Check sheet for the drawn part. Datum: minimum x, y, z corner. Units: mm. Coordinates: 2 decimals unless noted, no trailing zeros. Order: outer loops, then holes, each group sorted by start corner. A loop starts at its lowest first (then second) coordinate and runs counter-clockwise, first axis right, second up. Notation, with made-up numbers: (4.5, 30) - (41.5, 30) arc R24 ccw to (41.5, 50) - close; hole circle Ø1 at (-8, -13). An arc over 180 degrees is marked (long way). Answer as CSV lines item,"result". Start each with the question number.
1. Section check C-C (z = 0.65). Record the cut outline in (x, y) (1 decimal).
2. Go/stop test with a flat-tipped pin: pin 1 (4 mm diameter, centred on x = 33.655, y = 64.77, fed in from -Z). Record where the tip stops, or that it passes through.
3. Section check B-B (x = 33.5). Record the cut outline in (y, z).
4. Section check A-A (y = 24.13). Record the cut outline in (x, z).
5. Material ranges on L1, parallel to X at y = 153.67, z = 0.65; L2, parallel to Y at x = 32, z = 0.45; L3, parallel to Y at x = 15, z = 0.5 (1 decimal), recorded low to high. Write a range as [from, to].
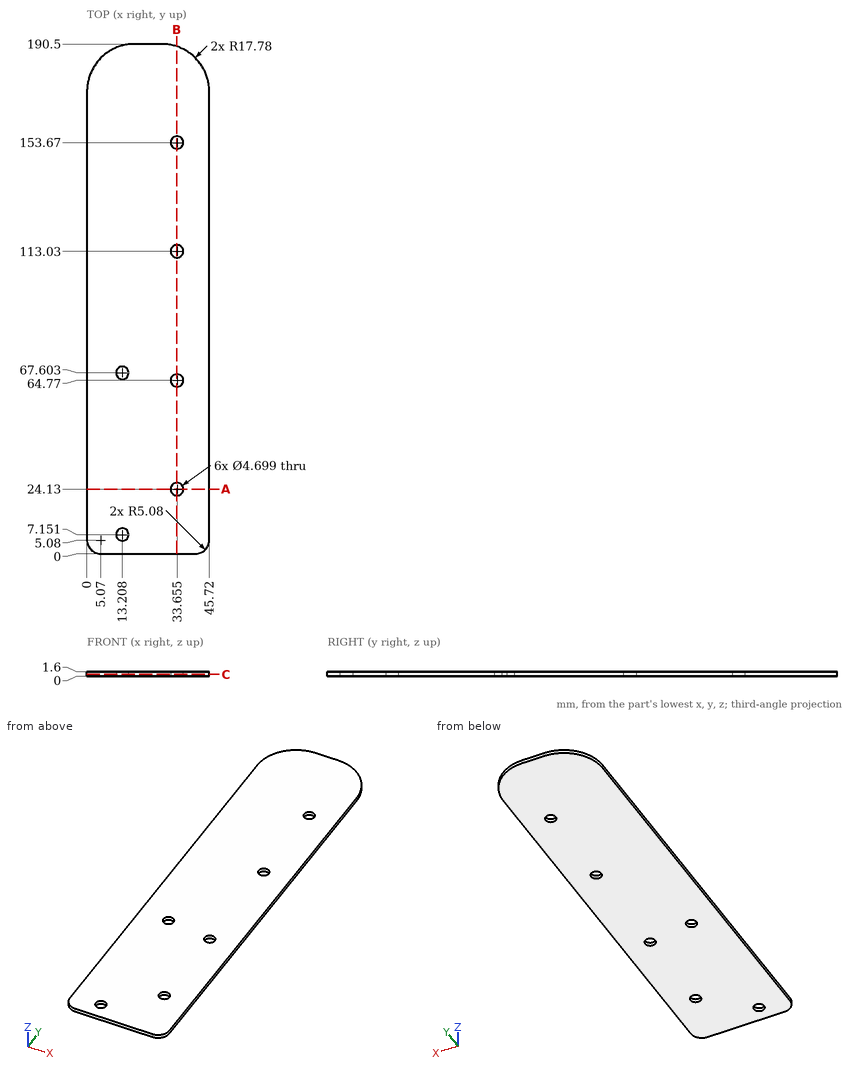
Evaluation:
1,outline,"(0, 4.8) arc R5.1 ccw to (5.1, 0) - (40.6, 0) arc R5.1 ccw to (45.7, 5.1) - (45.7, 172.7) arc R17.8 ccw to (27.9, 190.5) - (17.8, 190.5) arc R17.8 ccw to (0, 172.7) - close; hole circle Ø4.7 at (13.2, 7.2); hole circle Ø4.7 at (13.2, 67.6); hole circle Ø4.7 at (33.7, 24.1); hole circle Ø4.7 at (33.7, 64.8); hole circle Ø4.7 at (33.7, 113); hole circle Ø4.7 at (33.7, 153.7)"
2,pin 1,"passes through"
3,outline,"(0, 0) - (21.79, 0) - (21.79, 1.6) - (0, 1.6) - close; (26.47, 0) - (62.43, 0) - (62.43, 1.6) - (26.47, 1.6) - close; (67.11, 0) - (110.69, 0) - (110.69, 1.6) - (67.11, 1.6) - close; (115.37, 0) - (151.33, 0) - (151.33, 1.6) - (115.37, 1.6) - close; (156.01, 0) - (189.61, 0) - (189.61, 1.6) - (156.01, 1.6) - close"
4,outline,"(0, 0) - (31.31, 0) - (31.31, 1.6) - (0, 1.6) - close; (36, 0) - (45.72, 0) - (45.72, 1.6) - (36, 1.6) - close"
5,L1,"x = [0, 31.31], [36, 45.72]"
5,L2,"y = [0, 22.46], [25.8, 63.1], [66.44, 111.36], [114.7, 152], [155.34, 190.03]"
5,L3,"y = [0, 5.6], [8.7, 66.1], [69.1, 190.3]"
